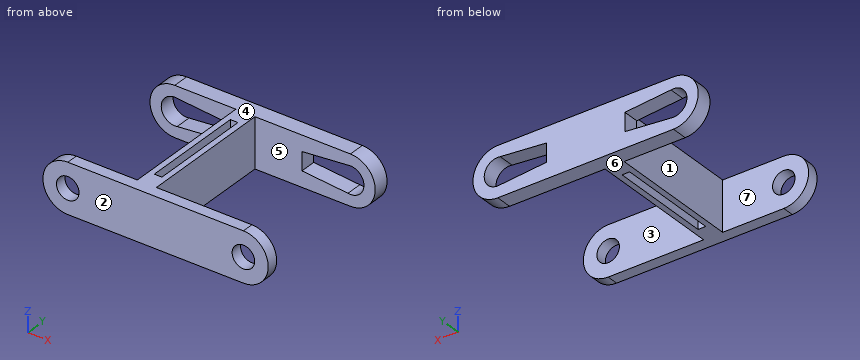
```python
from build123d import *

# Parameters (mm, degrees)
BOSS_EXTRUDE1_START   = 43.6
SKETCH1_R             = 6.5
BOSS_EXTRUDE1_DEPTH   = 2.1
BOSS_EXTRUDE1_2_DEPTH = 2.1
BOSS_EXTRUDE2_START   = 43.6
SKETCH2_W             = 46
SKETCH2_H             = 13
BOSS_EXTRUDE2_DEPTH   = 2.1
CUT_EXTRUDE1_START    = 43.6
SKETCH3_R             = 3.55
CUT_EXTRUDE1_DEPTH    = 2.1
CUT_EXTRUDE2_START    = 43.6
CUT_EXTRUDE2_DEPTH    = 2.1
BOSS_EXTRUDE3_START   = 5
SKETCH5_R             = 6.5
BOSS_EXTRUDE3_DEPTH   = 1.5
BOSS_EXTRUDE3_2_DEPTH = 1.5
BOSS_EXTRUDE4_START   = 5
SKETCH6_W             = 46
SKETCH6_H             = 13
BOSS_EXTRUDE4_DEPTH   = 1.5
CUT_EXTRUDE3_START    = 5
SKETCH7_R             = 2.95
CUT_EXTRUDE3_DEPTH    = 1.5
BOSS_EXTRUDE5_START   = 18.5
SKETCH8_W             = 13
SKETCH8_H             = 42.2
BOSS_EXTRUDE5_DEPTH   = 2.5
CUT_EXTRUDE4_START    = -0.01
SKETCH9_W             = 2
SKETCH9_H             = 27
CUT_EXTRUDE4_DEPTH    = 6.51


with BuildPart() as part:
    # Sketch1 → Boss-Extrude1 (new, symmetric)
    with BuildSketch(Plane(origin=(0, 0, 0), x_dir=(1, 0, 0), z_dir=(0, 1, 0)).offset(BOSS_EXTRUDE1_START)):
        with Locations(Location((0, 0, 0), (0, 0, 270))):
            Circle(SKETCH1_R)
    extrude(amount=BOSS_EXTRUDE1_DEPTH, both=True)



with BuildPart() as body_2:
    # Sketch1 → Boss-Extrude1 2 (new, symmetric)
    with BuildSketch(Plane(origin=(0, 0, 0), x_dir=(1, 0, 0), z_dir=(0, 1, 0)).offset(BOSS_EXTRUDE1_START)):
        with Locations(Location((46, 0, 0), (0, 0, 270))):
            Circle(SKETCH1_R)
    extrude(amount=BOSS_EXTRUDE1_2_DEPTH, both=True)


with BuildPart() as part_1:
    add(part.part)

    add(body_2.part)  # Boss-Extrude2 merges body 2
    # Sketch2 → Boss-Extrude2 (add, symmetric)
    with BuildSketch(Plane(origin=(0, 0, 0), x_dir=(1, 0, 0), z_dir=(0, 1, 0)).offset(BOSS_EXTRUDE2_START)):
        with Locations((23, 0)):
            Rectangle(SKETCH2_W, SKETCH2_H)
    extrude(amount=BOSS_EXTRUDE2_DEPTH, both=True)

    # Sketch3 → Cut-Extrude1 (cut, symmetric)
    with BuildSketch(Plane(origin=(0, 0, 0), x_dir=(1, 0, 0), z_dir=(0, 1, 0)).offset(CUT_EXTRUDE1_START)):
        with Locations(Location((0, 0, 0), (0, 0, 270))):
            Circle(SKETCH3_R)
        with Locations(Location((46, 0, 0), (0, 0, 270))):
            Circle(SKETCH3_R)
    extrude(amount=CUT_EXTRUDE1_DEPTH, both=True, mode=Mode.SUBTRACT)

    # Sketch4 → Cut-Extrude2 (cut, symmetric)
    with BuildSketch(Plane(origin=(0, 0, 0), x_dir=(1, 0, 0), z_dir=(0, 1, 0)).offset(CUT_EXTRUDE2_START)):
        Polygon((0, -3.55), (12.7, -2.403281405), (12.7, 2.403281405), (0, 3.55), align=None)
        Polygon((46, 3.55), (33.3, 2.403281405), (33.3, -2.403281405), (46, -3.55), align=None)
    extrude(amount=CUT_EXTRUDE2_DEPTH, both=True, mode=Mode.SUBTRACT)



with BuildPart() as body_2_2:
    # Sketch5 → Boss-Extrude3 (new, symmetric)
    with BuildSketch(Plane(origin=(0, 0, 0), x_dir=(1, 0, 0), z_dir=(0, 1, 0)).offset(BOSS_EXTRUDE3_START)):
        with Locations(Location((0, 0, 0), (0, 0, 270))):
            Circle(SKETCH5_R)
    extrude(amount=BOSS_EXTRUDE3_DEPTH, both=True)



with BuildPart() as body_3:
    # Sketch5 → Boss-Extrude3 2 (new, symmetric)
    with BuildSketch(Plane(origin=(0, 0, 0), x_dir=(1, 0, 0), z_dir=(0, 1, 0)).offset(BOSS_EXTRUDE3_START)):
        with Locations(Location((46, 0, 0), (0, 0, 270))):
            Circle(SKETCH5_R)
    extrude(amount=BOSS_EXTRUDE3_2_DEPTH, both=True)


with BuildPart() as body_2_2_1:
    add(body_2_2.part)

    add(body_3.part)  # Boss-Extrude4 merges body 3
    # Sketch6 → Boss-Extrude4 (add, symmetric)
    with BuildSketch(Plane(origin=(0, 0, 0), x_dir=(1, 0, 0), z_dir=(0, 1, 0)).offset(BOSS_EXTRUDE4_START)):
        with Locations((23, 0)):
            Rectangle(SKETCH6_W, SKETCH6_H)
    extrude(amount=BOSS_EXTRUDE4_DEPTH, both=True)

    # Sketch7 → Cut-Extrude3 (cut, symmetric)
    with BuildSketch(Plane(origin=(0, 0, 0), x_dir=(1, 0, 0), z_dir=(0, 1, 0)).offset(CUT_EXTRUDE3_START)):
        with Locations(Location((0, 0, 0), (0, 0, 270))):
            Circle(SKETCH7_R)
        with Locations(Location((46, 0, 0), (0, 0, 270))):
            Circle(SKETCH7_R)
    extrude(amount=CUT_EXTRUDE3_DEPTH, both=True, mode=Mode.SUBTRACT)


with BuildPart() as part_2:
    add(part_1.part)

    add(body_2_2_1.part)  # Boss-Extrude5 merges body 2 2
    # Sketch8 → Boss-Extrude5 (add, symmetric)
    with BuildSketch(Plane(origin=(0, 0, 0), x_dir=(0, 0, -1), z_dir=(1, 0, 0)).offset(BOSS_EXTRUDE5_START)):
        with Locations((0, 24.6)):
            Rectangle(SKETCH8_W, SKETCH8_H)
    extrude(amount=BOSS_EXTRUDE5_DEPTH, both=True)

    # Sketch9 → Cut-Extrude4 (cut, symmetric)
    with BuildSketch(Plane.XY.offset(CUT_EXTRUDE4_START)):
        with Locations((18.5, 24)):
            Rectangle(SKETCH9_W, SKETCH9_H)
    extrude(amount=CUT_EXTRUDE4_DEPTH, both=True, mode=Mode.SUBTRACT)


solid = part_2.part
```
Here's how the part is built. I have some questions about the finished solid (model axes, mm). Face numbers are marked on the shaded views. A direction names the side the tool comes from. Give positions to 0.01 mm unless a question says otherwise; leave off trailing zeros. Loops run counter-clockwise (first coordinate to the right, second up) from the corner with the lowest first, then second, coordinate; pieces in that order, holes last. Notation, with made-up numbers: (-8, 70.5) -> (7, 70.5) arc R36 cw to (7, 106.5) -> close; hole circle Ø2 at (9, 15). An arc over 180 degrees is marked (long way). Use one line per item in the form item = value. Start each with the question number.
1) Which directions (+Z, -Z, +X, -X, +Y, -Y) give clear straight access to the entire face, cutting with the end or side of a thin tool? Please do the marked faces 5, 6 and 7.
2) Imagine slicing it at A-A (x = 14). Please give me the cut outline in (y, z).
3) Please list where these lines run through material, in increasing order: line 1 along X through (y, z) = (5, 0); line 2 along X through (y, z) = (43.25, 0); line 3 along Y through (x, z) = (15, -4).
4) Imagine slicing it at C-C (y = 28.5). Please give me the cut outline in (x, z).
5) For P1, Ø12, axis at x = 38, y = 40, coming from the -Z side; P2, Ø4.5, axis at x = 46, z = 0, coming from the +Y side; P3, Ø5, axis at y = 27, z = 0, coming from the +X side; P4, Ø5, axis at y = 28.5, z = -5, coming from the -X side, each with a flat end and sliding along its axis, tell me the tip position at first contact or that it passes through.
6) Imagine slicing it at B-B (z = 0). Count the separate pieces of the cut face and the enclosed holes in it, then the cut area to 3 significant figures.
7) Imagine slicing it at D-D (x = 4). Please give me the cut outline in (y, z).
8) Thinking about a two-plate mould opening in Y: for the marked faces 1, 2, 3 and 4, which applies, +Y half, -Y half, draft (parallel to the pull), parting line (faces both ways), or undercut?
Check values:
q1.face_5 = +Z, -Z, +X
q1.face_6 = -Z, +X, -X, +Y, -Y
q1.face_7 = +Z, -Z, -X
q2.outline = (3.5, -6.5) -> (6.5, -6.5) -> (6.5, 6.5) -> (3.5, 6.5) -> close; (41.5, -6.5) -> (45.7, -6.5) -> (45.7, 6.5) -> (41.5, 6.5) -> close
q3.line_1 = -6.5 to -2.95, 2.95 to 43.05, 48.95 to 52.5
q3.line_2 = -6.5 to -3.55, 12.7 to 33.3, 49.55 to 52.5
q3.line_3 = 3.5 to 6.5, 41.5 to 45.7
q4.outline = (16, -6.5) -> (17.5, -6.5) -> (17.5, 6.5) -> (16, 6.5) -> close; (19.5, -6.5) -> (21, -6.5) -> (21, 6.5) -> (19.5, 6.5) -> close
q5.P1 = -6.5
q5.P2 = through
q5.P3 = 21
q5.P4 = 16
q6.separate_pieces = 5
q6.enclosed_holes = 1
q6.area = 374 mm^2
q7.outline = (3.5, -6.5) -> (6.5, -6.5) -> (6.5, 6.5) -> (3.5, 6.5) -> close; (41.5, -6.5) -> (45.7, -6.5) -> (45.7, -3.19) -> (41.5, -3.19) -> close; (41.5, 3.19) -> (45.7, 3.19) -> (45.7, 6.5) -> (41.5, 6.5) -> close
q8.face_1 = undercut
q8.face_2 = -Y half
q8.face_3 = undercut
q8.face_4 = draft
